Autodesk Inventor part; units mm, degrees
ref_plane "YZ Plane" through (0, 0, 0) normal (1, 0, 0) x (0, 1, 0)
ref_plane "XZ Plane" through (0, 0, 0) normal (0, 1, 0) x (-1, 0, 0)
ref_plane "XY Plane" through (0, 0, 0) normal (0, 0, 1) x (1, 0, 0)
sketch "Náčrt1" plane through (0, 0, 0) normal (0, 0, 1) x (1, 0, 0)
  line L0 (-24.5, 7.7937) -> (-24.5, -1.7063)
  line L1 (-24.5, -1.7063) -> (24.5, -1.7063)
  line L2 (24.5, -1.7063) -> (24.5, 7.7937)
  line L3 (24.5, 7.7937) -> (25, 7.7937)
  line L4 (25, 7.7937) -> (25, -2.2063)
  line L5 (25, -2.2063) -> (-25, -2.2063)
  line L6 (-25, -2.2063) -> (-25, 7.7937)
  line L7 (-25, 7.7937) -> (-24.5, 7.7937)
  point P0 (0, 0)
  point P1 (24.5, 3.0437)
  point P2 (-24.75, 7.7937)
  point P3 (24.75, 7.7937)
  dimension "d0" = 25
  dimension "d1" = 25
  dimension "d2" = 0.5
  dimension "d3" = 0.5
  dimension "d4" = 0.5
  dimension "d5" = 10
  dimension "d6" = 10
extrude "Vysunutí1" add sketch "Náčrt1" along normal blind 10
sketch "Náčrt2" plane through (25, -2.2063, 0) normal (1, 0, 0) x (0, 0, -1)
  circle A0 centre (-5, 5) radius 2
  line L0 (0, 0) -> (0, 10)
  point P0 (0, 2.2063)
  point P1 (0, 5)
  dimension "d9" = 4
  dimension "d10" = 5
extrude "Vysunutí2" cut sketch "Náčrt2" against normal through all
pattern_linear "Obdélníkové pole1" count 10 spacing 10 along (0, 0, 1) of "Vysunutí2"
sketch "Náčrt3" plane through (-24.5, -1.7063, 0) normal (0, 1, 0) x (1, 0, 0)
  circle A0 centre (4.5, -5) radius 2
  line L0 (49, -10) -> (0, -10)
  line L1 (-0.5, 0) -> (-0.5, -10)
  point P0 (24.5, 0)
  dimension "d16" = 4
  dimension "d17" = 5
  dimension "d18" = 5
extrude "Vysunutí3" cut sketch "Náčrt3" against normal through all
pattern_linear "Obdélníkové pole2" count 10 spacing 10 along (0, 0, -1) count 5 spacing 10 along (1, 0, 0) of "Vysunutí3"
sketch "Náčrt4" plane through (25, -2.2063, 0) normal (1, 0, 0) x (0, 0, -1)
  arc A0 (0, 5) -> (-10, 5) centre (-5, 5) ccw
  line L0 (0, 0) -> (0, 10)
  line L1 (0, 0) -> (-10, 0)
  line L2 (0, 10) -> (-10, 10)
  line L3 (-10, 10) -> (0, 10)
  line L4 (0, 10) -> (0, 5)
  line L5 (0, 10) -> (0, 0.5)
  line L6 (-10, 10) -> (-10, 0.5)
  line L7 (-10, 5) -> (-10, 10)
  point P0 (0, 2.2063)
  point P1 (-5, 10)
  dimension "d27" = 10
  dimension "d28" = 5
  dimension "d29" = 5
extrude "Vysunutí4" cut sketch "Náčrt4" against normal through all
fillet "Zaoblení1" radius 0.5 2 edges at (25, -2.2063, 5) (24.5, -1.7063, 5)
fillet "Zaoblení2" radius 0.5 2 edges at (-25, -2.2063, 5) (-24.5, -1.7063, 5)
properties part number "1031"
Part model, mm, in its own coordinate system. A direction names the side the tool comes from. Give positions to 0.01 mm unless a question says otherwise; leave off trailing zeros. Write each loop counter-clockwise with the first axis right and the second up, starting at its lowest first coordinate (ties: lowest second). Pieces come first, ordered by that corner, then holes. Notation, with made-up numbers: (26.5, -17) -> (85.5, -17) arc R38 ccw to (85.5, 21) -> close; hole circle Ø7 at (-38.75, 74). An arc over 180 degrees is marked (long way). Put each result on its own line as item: value. Start each with the question number.
Item 1: Cut at A-A (y = 0.25). List the corners of the cut face in (x, z), then the cut area to 3 significant figures.
Item 2: Cut at C-C (z = 4). State how many separate pieces and enclosed holes the cut face has, then the cut area to 3 significant figures.
Item 3: Pull direction X, two halves, no side cores. Call faces 3 (the face through (-24.5, 3.4, 2.7)), 4 (the face through (24.754, 7.792, 4.89)), 5 (the face through (-25, 0.87, 6.04)): pulls with the +X half, pulls with the -X half, needs draft (parallel to the pull), parting line crosses it, or undercut.
Item 4: Which spindle directions (+Z, -Z, +X, -X, +Y, -Y) get a long thin tool onto all of the face, cutting with end or side? Do faces 1 (the face through (24.5, 3.2, 2.7)), 2 (the face through (0, -2, 10)). Say none if no direction does.
Item 5: Pin check, flat tips, straight feed: pin 1 Ø2.5 at (y, z) = (2.79, 5) entering from -X; pin 2 Ø5 at (x, y) = (4.5, -0.5) entering from +Z; pin 3 Ø4.5 at (x, z) = (0, 5) entering from +Y. Stop position of each tip, or through.
Item 6: Cut at D-D (y = 3.75). List the corners of the cut face in (x, z).
Item 7: Cut at B-B (x = 20). List the corners of the cut face in (y, z).
Item 8: Wall check: L1, parallel to X at y = -1, z = 5.25; L2, parallel to X at y = -1.85, z = 5; L3, parallel to Z at x = 10, y = -1.9. Give the ranges that are in metal, low to high. Write a range as [from, to].
Answer list:
1. outline: (-25, 0) -> (-24.5, 0) -> (-24.5, 10) -> (-25, 10) -> close; (24.5, 0) -> (25, 0) -> (25, 10) -> (24.5, 10) -> close
1. area: 10.0 mm2
2. separate pieces: 8
2. enclosed holes: 0
2. area: 22.3 mm2
3. face 3: undercut
3. face 4: needs draft
3. face 5: pulls with the -X half
4. face 1: +Z, -Z, +Y
4. face 2: +Z, +X, -X, +Y, -Y
5. pin 1: passes through
5. pin 2: stops at z = 10
5. pin 3: stops at y = -1.71
6. outline: (-25, 0.09) -> (-24.5, 0.09) -> (-24.5, 3.24) -> (-25, 3.24) -> close; (-25, 6.76) -> (-24.5, 6.76) -> (-24.5, 9.91) -> (-25, 9.91) -> close; (24.5, 0.09) -> (25, 0.09) -> (25, 3.24) -> (24.5, 3.24) -> close; (24.5, 6.76) -> (25, 6.76) -> (25, 9.91) -> (24.5, 9.91) -> close
7. outline: (-2.21, 0) -> (-1.71, 0) -> (-1.71, 3) -> (-2.21, 3) -> close; (-2.21, 7) -> (-1.71, 7) -> (-1.71, 10) -> (-2.21, 10) -> close
8. L1: x = [-25, -24.5], [24.5, 25]
8. L2: x = [-24.98, -22], [-18, -12], [-8, -2], [2, 8], [12, 18], [22, 24.98]
8. L3: z = [0, 3], [7, 10]
